Drawing for the job (mm, zero at the part's lowest x, y, z). A direction names the side the tool comes from. Give positions to 0.01 mm unless a question says otherwise; leave off trailing zeros. Order: outer loops, then holes, each group sorted by start corner. A loop starts at its lowest first (then second) coordinate and runs counter-clockwise, first axis right, second up. Notation, with made-up numbers: (69, 73) - (98, 73) arc R29 ccw to (98, 103) - close; hole circle Ø11 at (42, -13.75). An arc over 180 degrees is marked (long way). Use a Markdown table: item, result.
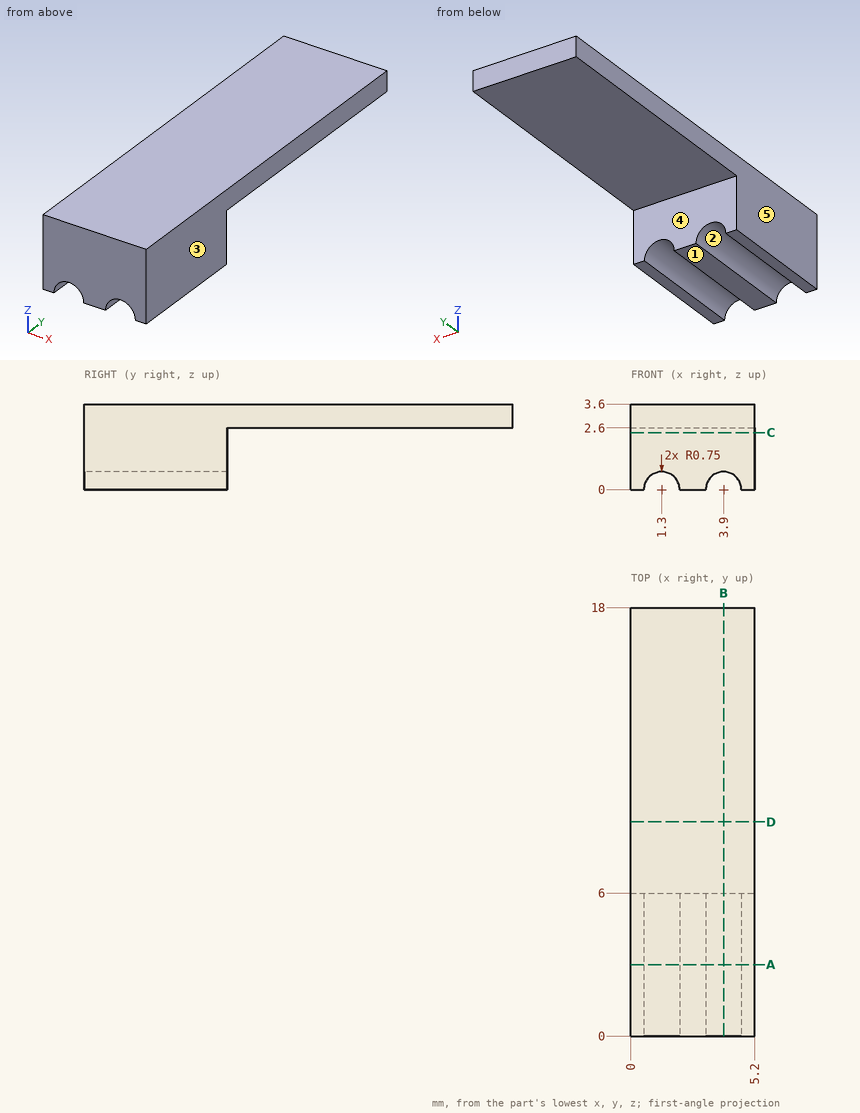
1) Slice it at D-D (y = 9). Write the cut outline in (x, z), and give its area (3 significant figures).
Computed:
| item | result |
|---|---|
| outline | (0, 2.6) - (5.2, 2.6) - (5.2, 3.6) - (0, 3.6) - close |
| area | 5.20 mm² |
2) Slice it at A-A (y = 3). Write the cut outline in (x, z).
Computed:
| item | result |
|---|---|
| outline | (0, 0) - (0.55, 0) arc R0.75 cw to (2.05, 0) - (3.15, 0) arc R0.75 cw to (4.65, 0) - (5.2, 0) - (5.2, 3.6) - (0, 3.6) - close |
3) Wall check: line 1 (Z direction, x = 2.5, y = 16.25); line 2 (Y direction, x = 4.65, z = 0.55). Give the ranges that are in metal, low to high. Write a range as from..to.
Computed:
| item | result |
|---|---|
| line 1 | z = 2.6..3.6 |
| line 2 | y = 0..6 |
4) Two-plate mould, pull along X, no slides. Class the marked faces 1, 2 and 3: +X half, -X half, draft (parallel to the pull), parting line (faces both ways), or undercut.
Computed:
| item | result |
|---|---|
| face 1 | draft |
| face 2 | undercut |
| face 3 | +X half |
5) Slice it at C-C (z = 2.4). Write the cut outline in (x, y).
Computed:
| item | result |
|---|---|
| outline | (0, 0) - (5.2, 0) - (5.2, 6) - (0, 6) - close |
6) Slice it at B-B (x = 3.9). Write the cut outline in (y, z).
Computed:
| item | result |
|---|---|
| outline | (0, 0.75) - (6, 0.75) - (6, 2.6) - (18, 2.6) - (18, 3.6) - (0, 3.6) - close |
7) Tool access for the marked faces 4 and 5: list every direction of +Z, -Z, +X, -X, +Y, -Y with a clear straight run to the whole face (end or side of a thin tool).
Computed:
| item | result |
|---|---|
| face 4 | -Z, +X, -X, +Y |
| face 5 | +Z, -Z, -X, +Y, -Y |
